Build history of the part. All positions in model axes, mm. Face numbers are marked on the shaded views. A direction names the side the tool comes from. Coordinates: 2 decimals unless noted, no trailing zeros. Write item = value, one per line. Start each with the question number.
Q1. Pull direction Z, two halves, no side cores. Call the marked faces 1 and 2: released by +Z, released by -Z, zero draft, split by the parting line, or undercut.
Q2. Pin check, flat tips, straight feed: P1, Ø1, axis at x = 6.5, y = -4, coming from the -Z side; P2, Ø2, axis at x = -4.5, y = -6.5, coming from the +Z side; P3, Ø0.5, axis at x = -2.5, y = 0.5, coming from the -Z side. Stop position of each tip, or through.
Q3. Drill centre lines: probe 1 along X at (y, z) = (0.1, 0); probe 2 along Y at (x, z) = (1.75, 0.25); probe 3 along Z at (x, y) = (0, 0.1). Where is each one in solid material? Low to high.
Q4. 3-axis set-ups, long thin cutter, end or side, ignore diameter. For the marked faces 3, 4, 5 and 6: which of +Z, -Z, +X, -X, +Y, -Y reach the whole face in a straight line?
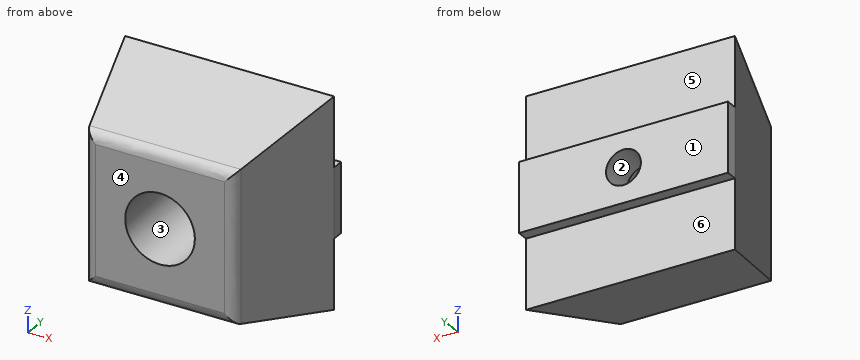
```python
from build123d import *

# Parameters (mm, degrees)
SKETCH1_W           = 18
SKETCH1_H           = 18
BOSS_EXTRUDE1_DEPTH = 10
BOSS_EXTRUDE1_TAPER = 15
SKETCH5_W           = 18
SKETCH5_H           = 6
BOSS_EXTRUDE3_DEPTH = 3
FILLET2_R           = 1
CUT_EXTRUDE3_REACH  = 15
SKETCH6_R           = 1.5
SKETCH7_R           = 3
CUT_EXTRUDE4_DEPTH  = 8
SKETCH9_W           = 20
SKETCH9_H           = 6
CUT_EXTRUDE5_DEPTH  = 2
FILLET4_R           = 1


with BuildPart() as part:
    # Sketch1 → Boss-Extrude1 (new body)
    with BuildSketch(Plane(origin=(0, 0, 0), x_dir=(1, 0, 0), z_dir=(0, 1, 0))):
        Rectangle(SKETCH1_W, SKETCH1_H)
    extrude(amount=-BOSS_EXTRUDE1_DEPTH, taper=BOSS_EXTRUDE1_TAPER)

    # Sketch5 → Boss-Extrude3 (add)
    with BuildSketch(Plane(origin=(0, 0, 0), x_dir=(1, 0, 0), z_dir=(0, 1, 0))):
        Rectangle(SKETCH5_W, SKETCH5_H)
    extrude(amount=BOSS_EXTRUDE3_DEPTH)

    # Fillet2
    fillet2_edges = [part.edges().sort_by_distance(p)[0] for p in [
        (0, 3, 3),
        (0, 3, -3),
    ]]
    fillet(fillet2_edges, radius=FILLET2_R)

    # Sketch6 → Cut-Extrude3 (cut, up to next)
    with BuildSketch(Plane(origin=(0, 3, 0), x_dir=(1, 0, 0), z_dir=(0, 1, 0)), mode=Mode.PRIVATE) as cut_extrude3_sk1:
        Circle(SKETCH6_R)
    cut_extrude3_tool1 = extrude(cut_extrude3_sk1.sketch, amount=-CUT_EXTRUDE3_REACH, mode=Mode.PRIVATE) & part.part
    add(cut_extrude3_tool1.solids().sort_by_distance((0, 3, 0))[0], mode=Mode.SUBTRACT)

    # Sketch7 → Cut-Extrude4 (cut)
    with BuildSketch(Plane.XZ.offset(10)):
        Circle(SKETCH7_R)
    extrude(amount=-CUT_EXTRUDE4_DEPTH, mode=Mode.SUBTRACT)

    # Sketch9 → Cut-Extrude5 (cut)
    with BuildSketch(Plane(origin=(0, 3, 0), x_dir=(1, 0, 0), z_dir=(0, 1, 0))):
        Rectangle(SKETCH9_W, SKETCH9_H)
    extrude(amount=-CUT_EXTRUDE5_DEPTH, mode=Mode.SUBTRACT)

    # Fillet4
    fillet4_edges = [part.edges().sort_by_distance(p)[0] for p in [
        (-6.320508076, -10, 0),
        (0, -10, 6.320508076),
        (6.320508076, -10, 0),
        (0, -10, -6.320508076),
    ]]
    fillet(fillet4_edges, radius=FILLET4_R)


solid = part.part
```
Recorded:
q1.face_1 = zero draft
q1.face_2 = undercut
q2.P1 = -8.06
q2.P2 = 7.53
q2.P3 = -3
q3.probe_1 = -9 to -1.5, 1.5 to 9
q3.probe_2 = -2 to 1
q3.probe_3 = -3 to -1.5, 1.5 to 3
q4.face_3 = -Y
q4.face_4 = +Z, -Z, +X, -X, -Y
q4.face_5 = +Z, +X, -X, +Y
q4.face_6 = -Z, +X, -X, +Y
